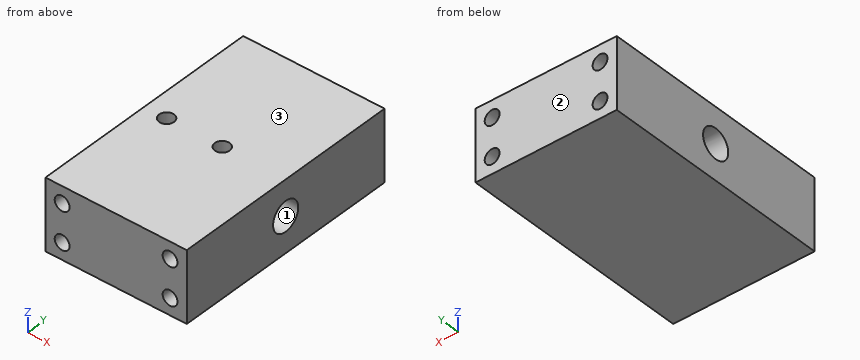
Autodesk Inventor part; units mm, degrees
ref_plane "YZ Plane" through (0, 0, 0) normal (1, 0, 0) x (0, 1, 0)
ref_plane "XZ Plane" through (0, 0, 0) normal (0, 1, 0) x (-1, 0, 0)
ref_plane "XY Plane" through (0, 0, 0) normal (0, 0, 1) x (1, 0, 0)
sketch "Sketch1" plane through (0, 0, 0) normal (0, 0, 1) x (1, 0, 0)
  line L0 (0, 0) -> (76.2, 0)
  line L1 (76.2, 0) -> (76.2, 125.8)
  line L2 (76.2, 125.8) -> (0, 125.8)
  line L3 (0, 125.8) -> (0, 0)
  circle A0 centre (12, 62.9) radius 4
  circle A1 centre (42, 62.9) radius 4
  dimension "d0" = 76.2
  dimension "d1" = 125.8
  dimension "d2" = 8
  dimension "d3" = 8
  dimension "d4" = 12
  dimension "d5" = 42
  dimension "d6" = 62.9
  dimension "d7" = 62.9
extrude "Extrusion1" add sketch "Sketch1" along normal blind 38.2 contours L3 L2 L1 L0 | A0 | A1
sketch "Sketch2" plane through (0, 0, 38.2) normal (0, 0, 1) x (1, 0, 0)
  line L0 (0, 0) -> (76.2, 0)
  line L1 (76.2, 0) -> (76.2, 125.8)
  line L2 (76.2, 125.8) -> (0, 125.8)
  line L3 (0, 125.8) -> (0, 0)
  circle A0 centre (12, 62.9) radius 4
  circle A1 centre (42, 62.9) radius 4
  dimension "d17" = 76.2
  dimension "d16" = 125.8
  dimension "d13" = 8
  dimension "d10" = 8
  dimension "d15" = 12
  dimension "d12" = 42
  dimension "d11" = 62.9
  dimension "d14" = 62.9
extrude "Extrusion2" cut sketch "Sketch2" against normal blind 19.1 contours A0 | A1
sketch "Sketch3" plane through (0, 0, 0) normal (-1, 0, 0) x (0, 0, 1)
  circle A0 centre (19.1, 62.9) radius 8
  line L0 (38.2, 125.8) -> (38.2, 0)
  line L1 (0, 0) -> (38.2, 0)
  dimension "d21" = 16
  dimension "d22" = 19.1
  dimension "d23" = 62.9
extrude "Extrusion3" cut sketch "Sketch3" against normal up to next
thread "Thread1"
thread "Thread2"
sketch "Sketch4" plane through (0, 0, 0) normal (0, -1, 0) x (1, 0, 0)
  circle A0 centre (9, 29.2) radius 4
  circle A1 centre (9, 9) radius 4
  circle A2 centre (67.2, 29.2) radius 4
  circle A3 centre (67.2, 9) radius 4
  line L0 (0, 38.2) -> (76.2, 38.2)
  line L1 (0, 0) -> (0, 38.2)
  dimension "d33" = 8
  dimension "d34" = 8
  dimension "d35" = 8
  dimension "d36" = 8
  dimension "d41" = 20.2
  dimension "d42" = 58.2
  dimension "d45" = 20.2
  dimension "d46" = 58.2
  dimension "d48" = 9
  dimension "d49" = 9
  dimension "d51" = 9
  dimension "d52" = 9
extrude "Extrusion4" cut sketch "Sketch4" against normal blind 30
sketch "Sketch5" plane through (0, 125.8, 38.2) normal (0, 1, 0) x (1, 0, 0)
  circle A0 centre (67.2, 29.2) radius 4
  circle A1 centre (67.2, 9) radius 4
  circle A2 centre (9, 29.2) radius 4
  circle A3 centre (9, 9) radius 4
  line L0 (0, 38.2) -> (76.2, 38.2)
  line L1 (0, 0) -> (0, 38.2)
  dimension "d56" = 8
  dimension "d55" = 8
  dimension "d64" = 8
  dimension "d63" = 8
  dimension "d65" = 20.2
  dimension "d59" = 58.2
  dimension "d58" = 20.2
  dimension "d62" = 58.2
  dimension "d61" = 9
  dimension "d66" = 9
  dimension "d60" = 9
  dimension "d57" = 9
extrude "Extrusion5" cut sketch "Sketch5" against normal blind 30
thread "Thread3"
thread "Thread4"
thread "Thread5"
thread "Thread6"
thread "Thread7"
thread "Thread8"
thread "Thread9"
thread "Thread10"
properties part number "MotorMountRight" material "Aluminum 6061"
Source: CAD feature listing. Evaluate the final solid. Frame: model axes, mm. Face numbers are marked on the shaded views. Round coordinates to 2 decimals unless told otherwise and drop trailing zeros. Loops run counter-clockwise (first coordinate to the right, second up) from the corner with the lowest first, then second, coordinate; pieces in that order, holes last. Notation, with made-up numbers: (44.25, 44.25) - (68.25, 44.25) arc R20 ccw to (68.25, 76.25) - close; hole circle Ø10 at (-39, 82.25). An arc over 180 degrees is marked (long way). Use CSV: the item, a comma, the result in double quotes.
Q1. Pin query (flat end, axial travel): pin 1 Ø8 at (y, z) = (32, 18) entering from -X; pin 2 Ø5 at (x, z) = (9, 29.2) entering from -Y; pin 3 Ø6.5 at (x, z) = (67.2, 9) entering from +Y. Return the tip coordinate at first contact, or that it passes through.
Reported:
pin 1,"x = 0"
pin 2,"y = 30"
pin 3,"y = 95.8"
Q2. Section query C-C, the plane y = 25. Output: boundary loops of the cut face in (x, z), then the cut area to 3 significant figures.
Reported:
outline,"(0, 0) - (76.2, 0) - (76.2, 38.2) - (0, 38.2) - close; hole circle Ø8 at (9, 9); hole circle Ø8 at (9, 29.2); hole circle Ø8 at (67.2, 9); hole circle Ø8 at (67.2, 29.2)"
area,"2,710 mm^2"
Q3. Mould query, pull axis Z, two halves, no side actions, for the marked faces 1, 2 and 3. Classes: pulls with the +Z half, pulls with the -Z half, needs draft (parallel to the pull), parting line crosses it, or undercut.
Reported:
face 1,"undercut"
face 2,"needs draft"
face 3,"pulls with the +Z half"
Q4. Section query D-D, the plane x = 42. Output: boundary loops of the cut face in (y, z), then the cut area to 3 significant figures.
Reported:
outline,"(0, 0) - (125.8, 0) - (125.8, 38.2) - (66.9, 38.2) - (66.9, 26.03) arc R8 cw (long way) to (58.9, 26.03) - (58.9, 38.2) - (0, 38.2) - close"
area,"4,510 mm^2"
Q5. Ray query, line 1 along X through (y, z) = (119.5, 9); line 2 along Z through (x, y) = (9, 115.25); line 3 along X through (y, z) = (62.9, 30). Return the intervals inside material, ascending.
Reported:
line 1,"0 to 5, 13 to 63.2, 71.2 to 76.2"
line 2,"0 to 5, 13 to 25.2, 33.2 to 38.2"
line 3,"0 to 8, 16 to 38, 46 to 76.2"
Q6. Section query A-A, the plane z = 19.5. Output: boundary loops of the cut face in (x, y).
Reported:
outline,"(0, 0) - (76.2, 0) - (76.2, 54.91) - (0, 54.91) - close; (0, 70.89) - (76.2, 70.89) - (76.2, 125.8) - (0, 125.8) - close"
Q7. Section query B-B, the plane x = 67.2. Output: boundary loops of the cut face in (y, z), then the cut area to 3 significant figures.
Reported:
outline,"(0, 0) - (125.8, 0) - (125.8, 5) - (95.8, 5) - (95.8, 13) - (125.8, 13) - (125.8, 25.2) - (95.8, 25.2) - (95.8, 33.2) - (125.8, 33.2) - (125.8, 38.2) - (0, 38.2) - (0, 33.2) - (30, 33.2) - (30, 25.2) - (0, 25.2) - (0, 13) - (30, 13) - (30, 5) - (0, 5) - close; hole circle Ø16 at (62.9, 19.1)"
area,"3,640 mm^2"
